Autodesk Inventor part; units mm, degrees
ref_plane "YZ Plane" through (0, 0, 0) normal (1, 0, 0) x (0, 1, 0)
ref_plane "XZ Plane" through (0, 0, 0) normal (0, 1, 0) x (-1, 0, 0)
ref_plane "XY Plane" through (0, 0, 0) normal (0, 0, 1) x (1, 0, 0)
sketch "Skizze1" plane through (0, 0, 0) normal (0, 0, 1) x (1, 0, 0)
  line L0 (-131.5, -112) -> (131.5, -112)
  line L1 (131.5, -112) -> (131.5, 112)
  line L2 (131.5, 112) -> (-131.5, 112)
  line L3 (-131.5, 112) -> (-131.5, -112)
  line L4 (-131.5, -112) -> (131.5, 112) construction
  line L5 (131.5, -112) -> (-131.5, 112) construction
  circle A0 centre (0, 102) radius 2.15
  line L6 (0, 156.8) -> (0, -156.8)
  circle A1 centre (-110, 102) radius 2.15
  circle A2 centre (110, 102) radius 2.15
  line L7 (-131.5, 0) -> (131.5, 0) construction
  circle A3 centre (0, -102) radius 2.15
  circle A4 centre (-110, -102) radius 2.15
  circle A5 centre (110, -102) radius 2.15
  point P0 (0, 0)
  dimension "d0" = 263
  dimension "d1" = 224
  dimension "d2" = 4.3
  dimension "d3" = 0
  dimension "d4" = 10
  dimension "d5" = 4.3
  dimension "d6" = 4.3
  dimension "d7" = 10
  dimension "d8" = 10
  dimension "d9" = 110
  dimension "d10" = 110
extrude "Grobblech1" add sketch "Skizze1" along normal blind 2 contours L3 L2 L6 A0 A3 L0 | L6 A3 A0 L2 L1 L0
fillet "Rundung1" radius 2 4 edges at (131.5, 112, 1) (131.5, -112, 1) (-131.5, -112, 1) (-131.5, 112, 1)
sketch "Skizze2" plane through (0, 0, 2) normal (0, 0, 1) x (1, 0, 0)
  arc A0 (-129.5, 112) -> (-131.5, 110) centre (-129.5, 110) ccw
  line L0 (-131.5, -110) -> (-131.5, 110)
  arc A1 (-131.5, -110) -> (-129.5, -112) centre (-129.5, -110) ccw
  line L1 (129.5, -112) -> (-129.5, -112)
  arc A2 (129.5, -112) -> (131.5, -110) centre (129.5, -110) ccw
  line L2 (131.5, 110) -> (131.5, -110)
  arc A3 (131.5, 110) -> (129.5, 112) centre (129.5, 110) ccw
  line L3 (-129.5, 112) -> (129.5, 112)
  circle A4 centre (110, -102) radius 2.15
  circle A5 centre (0, -102) radius 2.15
  circle A6 centre (-110, -102) radius 2.15
  circle A7 centre (110, 102) radius 2.15
  circle A8 centre (-110, 102) radius 2.15
  circle A9 centre (0, 102) radius 2.15
  line L4 (119.9374, -87) -> (-120.447, -87) construction
  line L5 (3.5, -87) -> (51.5, -87) construction
  line L6 (7, -90.5) -> (48, -90.5)
  line L7 (48, -83.5) -> (7, -83.5)
  arc A10 (7, -83.5) -> (7, -90.5) centre (7, -87) ccw
  arc A11 (48, -90.5) -> (48, -83.5) centre (48, -87) ccw
  line L8 (58.5, -87) -> (106.5, -87) construction
  line L9 (62, -90.5) -> (103, -90.5)
  line L10 (103, -83.5) -> (62, -83.5)
  arc A12 (62, -83.5) -> (62, -90.5) centre (62, -87) ccw
  arc A13 (103, -90.5) -> (103, -83.5) centre (103, -87) ccw
  line L11 (0, -102) -> (0, 102) construction
  line L12 (-327.71, -0.0001) -> (282.76, -0.0001) construction
  line L13 (-3.5, -87) -> (-51.5, -87) construction
  line L14 (-7, -90.5) -> (-48, -90.5)
  line L15 (-48, -83.5) -> (-7, -83.5)
  arc A14 (-7, -90.5) -> (-7, -83.5) centre (-7, -87) ccw
  arc A15 (-48, -83.5) -> (-48, -90.5) centre (-48, -87) ccw
  arc A16 (-62, -90.5) -> (-62, -83.5) centre (-62, -87) ccw
  line L16 (-62, -90.5) -> (-103, -90.5)
  line L17 (-103, -83.5) -> (-62, -83.5)
  line L18 (-58.5, -87) -> (-106.5, -87) construction
  arc A17 (-103, -83.5) -> (-103, -90.5) centre (-103, -87) ccw
  line L19 (3.5, 86.9998) -> (51.5, 86.9998) construction
  line L20 (7, 90.4998) -> (48, 90.4998)
  line L21 (48, 83.4998) -> (7, 83.4998)
  arc A18 (7, 90.4998) -> (7, 83.4998) centre (7, 86.9998) ccw
  arc A19 (48, 83.4998) -> (48, 90.4998) centre (48, 86.9998) ccw
  arc A20 (62, 90.4998) -> (62, 83.4998) centre (62, 86.9998) ccw
  line L22 (62, 90.4998) -> (103, 90.4998)
  line L23 (103, 83.4998) -> (62, 83.4998)
  line L24 (58.5, 86.9998) -> (106.5, 86.9998) construction
  arc A21 (103, 83.4998) -> (103, 90.4998) centre (103, 86.9998) ccw
  line L25 (-3.5, 86.9998) -> (-51.5, 86.9998) construction
  line L26 (-58.5, 86.9998) -> (-106.5, 86.9998) construction
  line L27 (-7, 90.4998) -> (-48, 90.4998)
  line L28 (-62, 90.4998) -> (-103, 90.4998)
  arc A22 (-7, 83.4998) -> (-7, 90.4998) centre (-7, 86.9998) ccw
  line L29 (-48, 83.4998) -> (-7, 83.4998)
  arc A23 (-48, 90.4998) -> (-48, 83.4998) centre (-48, 86.9998) ccw
  arc A24 (-62, 83.4998) -> (-62, 90.4998) centre (-62, 86.9998) ccw
  line L30 (-103, 83.4998) -> (-62, 83.4998)
  arc A25 (-103, 90.4998) -> (-103, 83.4998) centre (-103, 86.9998) ccw
  point P0 (0, 0)
  point P1 (65.6161, -112)
  point P2 (15.6161, -112)
  point P3 (-15.6161, -112)
  point P4 (-65.6161, -112)
  point P5 (5.6161, -112)
  point P6 (-5.6161, -112)
  point P7 (27.5, -87)
  point P8 (82.5, -87)
  point P9 (-119.9374, -87)
  point P10 (-27.5, -87)
  point P11 (-82.5, -87)
  point P12 (27.5, 86.9998)
  point P13 (82.5, 86.9998)
  point P14 (-27.5, 86.9998)
  point P15 (-82.5, 86.9998)
  dimension "d13" = 25
  dimension "d14" = 110
  dimension "d15" = 48
  dimension "d16" = 7
  dimension "d17" = 3.5
  dimension "d18" = 48
  dimension "d19" = 7
  dimension "d20" = 7
  dimension "d21" = 3.5
extrude "Extrusion1" cut sketch "Skizze2" against normal blind 10 contours A10 L7 A11 L6 | A12 L10 A13 L9 | L14 A15 L15 A14 | L16 A17 L17 A16 | L20 A19 L21 A18 | L22 A21 L23 A20 | A22 L29 A23 L27 | A24 L30 A25 L28
equation "\"d5\" = d2"
equation "\"d6\" = d2"
equation "\"d7\" = d4"
equation "\"d8\" = d4"
equation "\"d11\" = Stärke"
equation "\"Biegeradius\" = Stärke"
equation "\"BreiteBiegungsfreistellung\" = Stärke"
equation "\"TiefeBiegungsfreistellung\" = 0.5 * Stärke"
equation "\"GrößeEckenfreistellung\" = 4 * Stärke"
equation "\"MinimalRest\" = 2 * Stärke"
equation "\"Übergangsradius\" = Biegeradius"
equation "\"JacobiRadiusGröße\" = Biegeradius"
equation "\"Abstandsgröße\" = Stärke"
properties part number "Deckel"
Check sheet for the modelled part. Datum: model origin and axes. Units: mm. Round coordinates to 2 decimals unless told otherwise and drop trailing zeros. Order: outer loops, then holes, each group sorted by start corner. A loop starts at its lowest first (then second) coordinate and runs counter-clockwise, first axis right, second up. Notation, with made-up numbers: M 33.25,-23.75 L 62.25,-23.75 A21 ccw 62.25,-15.75 Z; hole C -37,41.25 d2. An arc over 180 degrees is marked long. One line per item, written item: value. Start each with the question number.
1. Gauge pin test, flat ends, axial feed: P1, Ø7, axis at x = -110, y = 102, coming from the +Z side; P2, Ø3, axis at x = 76, y = -88, coming from the +Z side. Record the tip position at first contact, or that the pin passes through.
2. Scan lines: line 1 along Y through (x, z) = (82.5, 1.35); line 2 along Y through (x, z) = (-110, 1.5); line 3 along X through (y, z) = (88.5, 1.1). Record each from-to range of solid material in increasing order.
3. Section check A-A on x = -72. Enter the section's corners in (y, z), and give its area (3 significant figures).
4. Section check B-B on z = 0.75. Give the number of separate pieces and of enclosed holes in the cut face, and give its area (3 significant figures).
Results found:
1. P1: z = 2
1. P2: through
2. line 1: -112 to -90.5, -83.5 to 83.5, 90.5 to 112
2. line 2: -112 to -104.15, -99.85 to 99.85, 104.15 to 112
2. line 3: -131.5 to -106.16, -58.84 to -51.16, -3.84 to 3.84, 51.16 to 58.84, 106.16 to 131.5
3. outline: M -112,0 L -90.5,0 L -90.5,2 L -112,2 Z; M -83.5,0 L 83.5,0 L 83.5,2 L -83.5,2 Z; M 90.5,0 L 112,0 L 112,2 L 90.5,2 Z
3. area: 420 mm^2
4. separate pieces: 1
4. enclosed holes: 14
4. area: 56,200 mm^2
